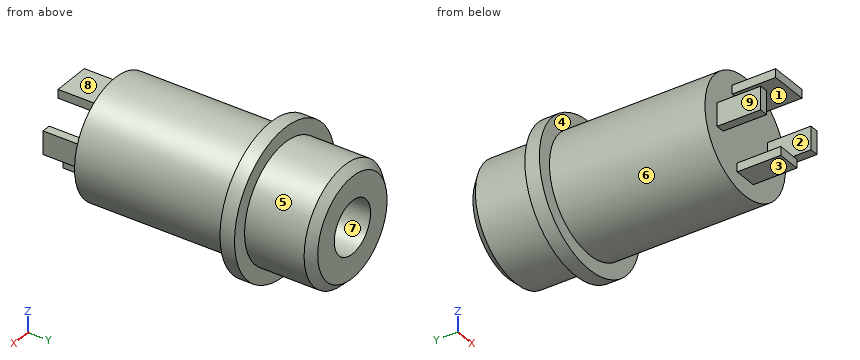
from build123d import *

# Parameters (mm, degrees)
SKETCH1_R           = 4
SKETCH1_R_2         = 1.8
SKETCH1_W           = 1.6
SKETCH1_H           = 0.6
SKETCH1_W_2         = 0.6
SKETCH1_H_2         = 1.6
SKETCH1_W_3         = 2.6
BOSS_EXTRUDE1_DEPTH = 11.7
SKETCH1_3_R         = 5
SKETCH1_3_R_2       = 4
BOSS_EXTRUDE2_DEPTH = 1
CUT_EXTRUDE1_START  = 4.65
SKETCH1_7_R         = 1.8
CUT_EXTRUDE1_DEPTH  = 15.2
BOSS_EXTRUDE5_START = -11.7
SKETCH1_8_W         = 0.6
SKETCH1_8_H         = 1.6
SKETCH1_8_W_2       = 1.6
SKETCH1_8_H_2       = 0.6
SKETCH1_8_W_3       = 2.6
BOSS_EXTRUDE5_DEPTH = 3


# Read off the part's stored shape, not the designer's step: M8x1.0 Machine Threads Stud3
with BuildPart() as part:
    # Sketch1 → Boss-Extrude1 (new body)
    with BuildSketch(Plane(origin=(0, 0, 0), x_dir=(1, 0, 0), z_dir=(0, 1, 0))):
        with Locations(Location((0, 0, 0), (0, 0, 270))):
            Circle(SKETCH1_R)
        Circle(SKETCH1_R_2)
        with Locations((0, 2.5)):
            Rectangle(SKETCH1_W, SKETCH1_H)
        with Locations((2.5, 0)):
            Rectangle(SKETCH1_W_2, SKETCH1_H_2)
        with Locations((0, -2.5)):
            Rectangle(SKETCH1_W_3, SKETCH1_H)
        with Locations((-2.5, 0)):
            Rectangle(SKETCH1_W_2, SKETCH1_H_2)
    extrude(amount=-BOSS_EXTRUDE1_DEPTH)

    # Sketch1<3> → Boss-Extrude2 (add)
    with BuildSketch(Plane(origin=(0, 0, 0), x_dir=(1, 0, 0), z_dir=(0, 1, 0))):
        with Locations(Location((0, 0, 0), (0, 0, 270))):
            Circle(SKETCH1_3_R)
        with Locations(Location((0, 0, 0), (0, 0, 270))):
            Circle(SKETCH1_3_R_2, mode=Mode.SUBTRACT)
    extrude(amount=-BOSS_EXTRUDE2_DEPTH)

    # M8x1.0 Machine Threads Stud3 outline → M8x1.0 Machine Threads Stud3 (revolve)
    with BuildSketch(Plane.XY):
        Polygon((4, 0), (4, 4.0955), (3.4455, 4.65), (0, 4.65), (0, 0), align=None)
    revolve(axis=Axis((0, 0, 0), (0, 1, 0)))

    # Sketch1<7> → Cut-Extrude1 (cut)
    with BuildSketch(Plane(origin=(0, 0, 0), x_dir=(1, 0, 0), z_dir=(0, 1, 0)).offset(CUT_EXTRUDE1_START)):
        with Locations(Location((0, 0, 0), (0, 0, 270))):
            Circle(SKETCH1_7_R)
    extrude(amount=-CUT_EXTRUDE1_DEPTH, mode=Mode.SUBTRACT)

    # Sketch1<8> → Boss-Extrude5 (add)
    with BuildSketch(Plane(origin=(0, 0, 0), x_dir=(1, 0, 0), z_dir=(0, 1, 0)).offset(BOSS_EXTRUDE5_START)):
        with Locations((2.5, 0)):
            Rectangle(SKETCH1_8_W, SKETCH1_8_H)
        with Locations((0, 2.5)):
            Rectangle(SKETCH1_8_W_2, SKETCH1_8_H_2)
        with Locations((-2.5, 0)):
            Rectangle(SKETCH1_8_W, SKETCH1_8_H)
        with Locations((0, -2.5)):
            Rectangle(SKETCH1_8_W_3, SKETCH1_8_H_2)
    extrude(amount=-BOSS_EXTRUDE5_DEPTH)


solid = part.part
Check sheet for the modelled part. Datum: model origin and axes. Units: mm. Face numbers are marked on the shaded views. A direction names the side the tool comes from. Round coordinates to 2 decimals unless told otherwise and drop trailing zeros. Order: outer loops, then holes, each group sorted by start corner. A loop starts at its lowest first (then second) coordinate and runs counter-clockwise, first axis right, second up.
(1) Cross-section at C-C, the plane y = -5.75. Enter the section's corners in (x, z), and give its area (3 significant figures).
(2) Scan lines: probe 1 along X at (y, z) = (-5, 0); probe 2 along Y at (x, z) = (-0.75, -0.5); probe 3 along Y at (x, z) = (-2, -1.25). Record each from-to range of solid material in increasing order.
(3) Go/stop test with flat-tipped pins: P1, Ø0.7, axis at x = -2.5, y = -13, coming from the -Z side; P2, Ø1.3, axis at x = 0, y = -13, coming from the +Z side; P3, Ø1.5, axis at y = 1, z = -4, coming from the +X side. Record where each tip stops, or that it passes through.
(4) Cross-section at B-B, the plane x = 0. Enter the section's corners in (y, z).
(5) Draft check along X on the marked faces 6, 7, 8 and 9. Enter one of: pulls with the +X half, pulls with the -X half, needs draft (parallel to the pull), parting line crosses it, or undercut.
(6) Cross-section at A-A, the plane z = 0. Enter the section's corners in (x, y), and give its area (3 significant figures).
(7) Access from +Z, -Z, +X, -X, +Y, -Y to the whole of each face (thin tool, end or side, straight path). Record for the marked faces 1, 2, 3, 4 and 5.
Check sheet entries:
1. outline: circle Ø8 at (0, 0); hole circle Ø3.6 at (0, 0)
1. area: 40.1 mm2
2. probe 1: x = -4 to -1.8, 1.8 to 4
2. probe 2: y = -11.7 to -10.55
2. probe 3: y = -11.7 to 4.65
3. P1: stops at z = -0.8
3. P2: stops at z = 2.8
3. P3: stops at x = 2.33
4. outline: (-14.7, -2.8) - (-11.7, -2.8) - (-11.7, -4) - (-1, -4) - (-1, -5) - (0, -5) - (0, -4) - (4.1, -4) - (4.65, -3.45) - (4.65, -1.8) - (-10.55, -1.8) - (-10.55, 1.8) - (4.65, 1.8) - (4.65, 3.45) - (4.1, 4) - (0, 4) - (0, 5) - (-1, 5) - (-1, 4) - (-11.7, 4) - (-11.7, 2.8) - (-14.7, 2.8) - (-14.7, 2.2) - (-11.7, 2.2) - (-11.7, -2.2) - (-14.7, -2.2) - close
5. face 6: parting line crosses it
5. face 7: undercut
5. face 8: needs draft
5. face 9: pulls with the -X half
6. outline: (-5, -1) - (-4, -1) - (-4, -11.7) - (-2.8, -11.7) - (-2.8, -14.7) - (-2.2, -14.7) - (-2.2, -11.7) - (2.2, -11.7) - (2.2, -14.7) - (2.8, -14.7) - (2.8, -11.7) - (4, -11.7) - (4, -1) - (5, -1) - (5, 0) - (4, 0) - (4, 4.1) - (3.45, 4.65) - (1.8, 4.65) - (1.8, -10.55) - (-1.8, -10.55) - (-1.8, 4.65) - (-3.45, 4.65) - (-4, 4.1) - (-4, 0) - (-5, 0) - close
6. area: 81.4 mm2
7. face 1: +X, -X, -Y
7. face 2: +Z, -Z, -Y
7. face 3: -Z, +X, -X, -Y
7. face 4: -Y
7. face 5: +Y
